Input: dimensioned drawing with shaded views. Units: mm. Origin: part minimum x, y, z. A direction names the side the tool comes from. Round coordinates to 2 decimals unless told otherwise and drop trailing zeros. Loops run counter-clockwise (first coordinate to the right, second up) from the corner with the lowest first, then second, coordinate; pieces in that order, holes last. Notation, with made-up numbers: (-37, 10.5) - (6, 10.5) arc R14 ccw to (6, 31.5) - close; hole circle Ø8 at (67, 33). An arc over 180 degrees is marked (long way). Use CSV: the item, a comma, the result in double quotes. Start each with the question number.
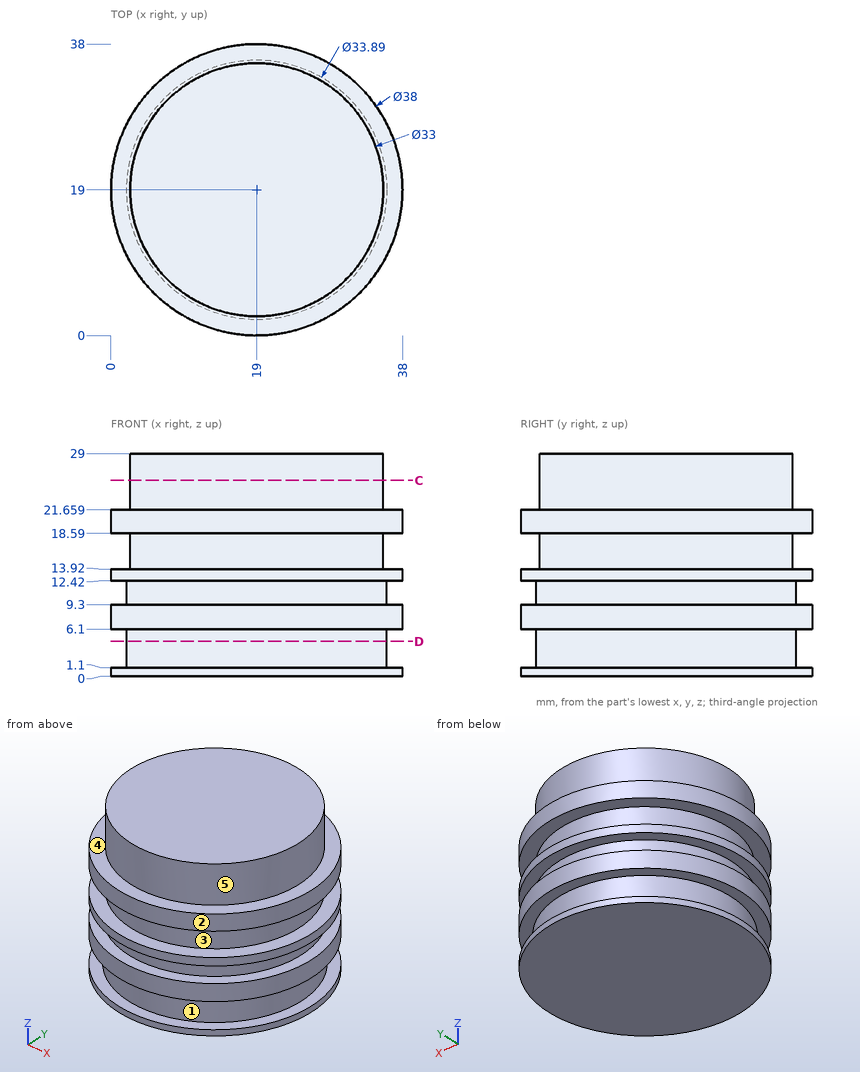
1. Line query: line 1 along Z through (x, y) = (10, 34); line 2 along X through (y, z) = (18.5, 20.5); line 3 along X through (y, z) = (11, 23). Output: solid intervals per line, ascending.
2. Contact query for flat-ended pins moving along their axis: P1, Ø10, axis at x = 32, z = 12.5, coming from the -Y side; P2, Ø1.5, axis at x = 15.5, z = 25, coming from the +Y side; P3, Ø6, axis at x = 25, z = 17, coming from the +Y side. Output: stop coordinate, or through.
3. Section query D-D on z = 4.5. Return the cut outline in (x, y) (1 decimal), and give its area (3 significant figures).
4. Reachability of the marked faces 1 and 2 from +Z, -Z, +X, -X, +Y, -Y: full face, straight path, thin tool, end or side. Return the list, or none.
5. Mould query, pull axis Z, two halves, no side actions, for the marked faces 3, 4 and 5. Classes: +Z half, -Z half, draft (parallel to the pull), parting line (faces both ways), or undercut.
6. Section query C-C on z = 25.5. Return the cut outline in (x, y), and give its area (3 significant figures).
Values:
1,line 1,"z = 0 to 1.1, 6.1 to 9.3, 12.42 to 13.92, 18.59 to 21.66"
1,line 2,"x = 0.01 to 37.99"
1,line 3,"x = 4.57 to 33.43"
2,P1,"stops at y = 1.77"
2,P2,"stops at y = 35.27"
2,P3,"stops at y = 37.68"
3,outline,"circle Ø33.9 at (19, 19)"
3,area,"902 mm^2"
4,face 1,"none"
4,face 2,"+Z, -Z"
5,face 3,"undercut"
5,face 4,"+Z half"
5,face 5,"draft"
6,outline,"circle Ø33 at (19, 19)"
6,area,"855 mm^2"
